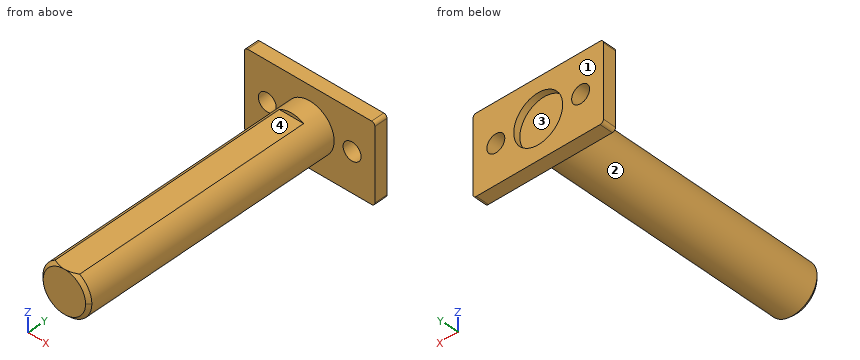
```python
from build123d import *

# Parameters (mm, degrees)
F0_W      = 40
F0_H      = 24
F0_R      = 7.5
F1_DEPTH  = 4
F2_DEPTH  = 85
F4_D      = 5.5
F6_DEPTH  = 75
F7_R      = 1
F8_SIZE2  = 0.99999
F8_SIZE   = 0.99999
F9_R      = 7.5
F10_DEPTH = 2


# Not quite as in the source:
# - a fillet or chamfer is up to 0.001 mm smaller than in the source, because OpenCascade refuses the exact size


with BuildPart() as f1:
    # F0 (on Front) → F1 (new body)
    with BuildSketch(Plane.XZ):
        Rectangle(F0_W, F0_H)
        Circle(F0_R, mode=Mode.SUBTRACT)
    extrude(amount=F1_DEPTH)

    # F0 (on Front) → F2 (join)
    with BuildSketch(Plane.XZ):
        Circle(F0_R)
    extrude(amount=F2_DEPTH)

    # F4 (through all)
    with Locations(Plane.XZ.offset(4)):
        with Locations((-13, 0), (13, 0)):
            Hole(F4_D / 2)

    # F5 (on face) → F6 (cut)
    with BuildSketch(Plane.XZ.offset(85)):
        with BuildLine():
            Line((8.4905531257, 12.6322833821), (-12.126554407, 6.5))
            Line((-12.126554407, 6.5), (-3.7416573868, 6.5))
            ThreePointArc((-3.7416573868, 6.5), (0, 7.5), (3.7416573868, 6.5))
            Line((3.7416573868, 6.5), (18.1320688201, 6.5))
            Line((18.1320688201, 6.5), (8.4905531257, 12.6322833821))
        make_face()
        with BuildLine():
            ThreePointArc((3.7416573868, 6.5), (0, 7.5), (-3.7416573868, 6.5))
            Line((-3.7416573868, 6.5), (3.7416573868, 6.5))
        make_face()
    extrude(amount=-F6_DEPTH, mode=Mode.SUBTRACT)

    # F7
    f7_edges = [f1.edges().sort_by_distance(p)[0] for p in [
        (-20, -2, 12),
        (20, -2, 12),
        (20, -2, -12),
        (-20, -2, -12),
    ]]
    fillet(f7_edges, radius=F7_R)

    # F8 (size 1 and 1 in the source; OpenCascade refuses exactly that, so slightly less here)
    f8_edges = [f1.edges().sort_by_distance(p)[0] for p in [
        (-3.754169, -85, -6.492782),
        (6.492782, -85, 3.754169),
    ]]
    chamfer(f8_edges, length=F8_SIZE, length2=F8_SIZE2)

    # F9 (on face) → F10 (cut)
    with BuildSketch(Plane(origin=(0, 0, 0), x_dir=(-1, 0, 0), z_dir=(0, 1, 0))):
        Circle(F9_R)
    extrude(amount=-F10_DEPTH, mode=Mode.SUBTRACT)


solid = f1.part
```
Geometry check sheet. Reference: the model listing, model coordinates, mm. Face numbers are marked on the shaded views. Give positions to 0.01 mm unless a question says otherwise; leave off trailing zeros. Loops run counter-clockwise (first coordinate to the right, second up) from the corner with the lowest first, then second, coordinate; pieces in that order, holes last. Notation, with made-up numbers: M 53.25,-23.5 L 80.25,-23.5 A17 ccw 80.25,7.5 Z; hole C 88.25,-30 d1. An arc over 180 degrees is marked long. Write item = value, one per line. Start each with the question number.
1. Section check A-A, the plane x = 13. Enter the section's corners in (y, z).
2. Thickness scan on probe 1 along Z at (x, y) = (13, -1); probe 2 along Z at (x, y) = (0, -1.1); probe 3 along Y at (x, z) = (8, -10). Record the ranges inside material, lowest first.
3. Section check C-C, the plane z = -1.5. Give the number of separate pieces and of enclosed holes in the cut face, plus the area to 3 significant figures.
4. Go/stop test with flat-tipped pins: P1, Ø7, axis at x = -13, z = 0, coming from the -Y side; P2, Ø10, axis at y = -44, z = 2.5, coming from the +X side; P3, Ø2, axis at y = -65.5, z = 2.5, coming from the +X side. Record where each tip stops, or that it passes through.
5. Draft check along Z on the marked faces 1, 2, 3 and 4. Enter one of: +Z half, -Z half, draft (parallel to the pull), parting line (faces both ways), or undercut.
6. Section check B-B, the plane y = -12.5. Enter the section's corners in (x, z), plus the area to 3 significant figures.
Values follow:
q1.outline = M -4,-12 L 0,-12 L 0,-2.75 L -4,-2.75 Z; M -4,2.75 L 0,2.75 L 0,12 L -4,12 Z
q2.probe_1 = -12 to -2.75, 2.75 to 12
q2.probe_2 = -12 to -7.5, 7.5 to 12
q2.probe_3 = -4 to 0
q3.separate_pieces = 3
q3.enclosed_holes = 0
q3.area = 1,280 mm^2
q4.P1 = -4
q4.P2 = 7.5
q4.P3 = 7.35
q5.face_1 = draft
q5.face_2 = parting line
q5.face_3 = undercut
q5.face_4 = +Z half
q6.outline = M -3.74,6.5 A7.5 ccw long 3.74,6.5 Z
q6.area = 172 mm^2
